The drawing under review shows one solid part. Ordinate dimensions are in mm from its lowest x, y, z. A direction names the side the tool comes from. Coordinates: 2 decimals unless noted, no trailing zeros. Write each loop counter-clockwise with the first axis right and the second up, starting at its lowest first coordinate (ties: lowest second). Pieces come first, ordered by that corner, then holes. Notation, with made-up numbers: M 75.25,15.5 L 90.25,15.5 A20 cw 90.25,54.5 Z; hole C 1,60.5 d9. An arc over 180 degrees is marked long. Write item = value, one per line.
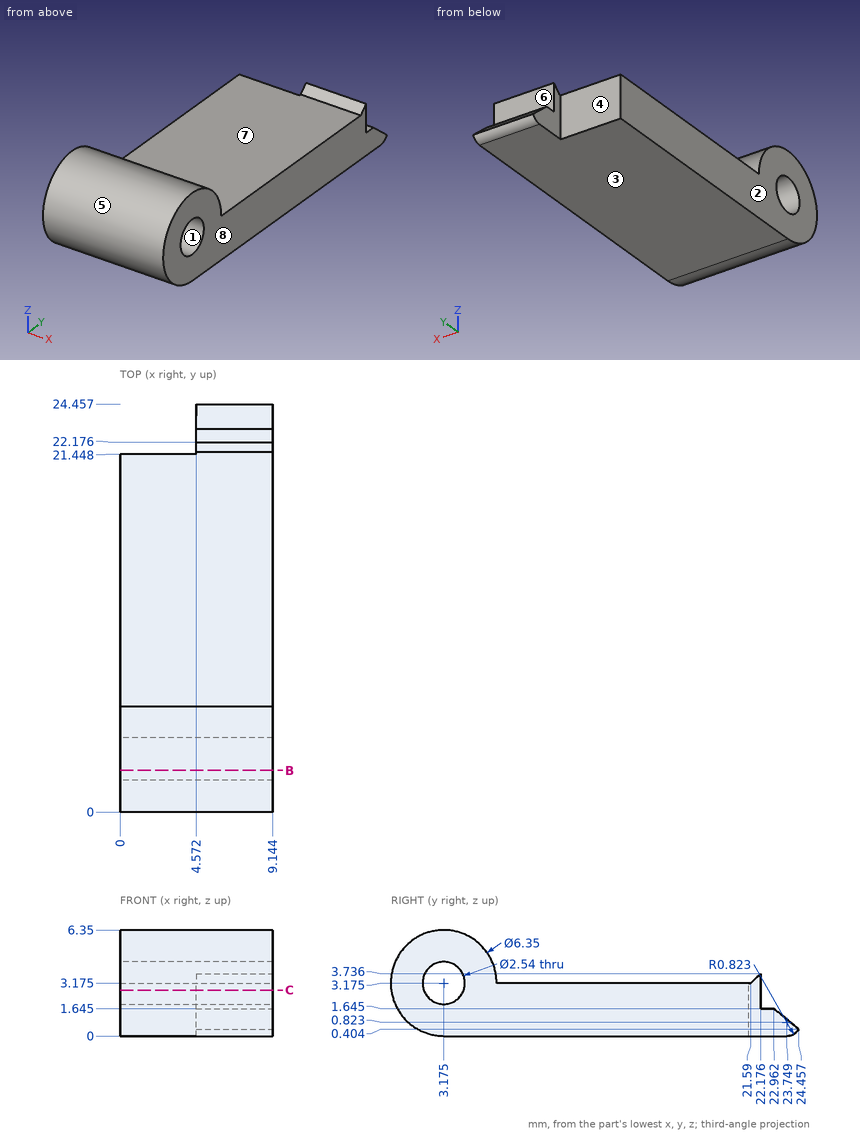
Q1. The part is to be moulded in two halves that separate along Z. For the marked faces 1, 2 and 3, say which applies: +Z half, -Z half, draft (parallel to the pull), parting line (faces both ways), or undercut.
Check result:
face_1 = undercut
face_2 = draft
face_3 = -Z half
Q2. Wall thickness on line 1 (X direction, y = 21.5, z = 1.25); line 2 (Z direction, x = 4.25, y = 13) (1 decimal); line 3 (Y direction, x = 7, z = 5.5) (1 decimal): over which ranges is each line inside the solid? List them lowest first.
Check result:
line_1 = 4.57 to 9.14
line_2 = 0 to 3.2
line_3 = 1 to 5.3
Q3. Consider section B-B, the plane y = 2.5. State the section outline as (x, z) points.
Check result:
outline = M 0,0.07 L 9.14,0.07 L 9.14,2.1 L 0,2.1 Z; M 0,4.25 L 9.14,4.25 L 9.14,6.28 L 0,6.28 Z
Q4. Machinability: for the marked faces 4, 5, 6, 7 and 8, which of the approach directions +Z, -Z, +X, -X, +Y, -Y give a long, thin tool a straight path to every point of the face, cutting with its end or side? Answer none if there is none.
Check result:
face_4 = +Z, -Z, -X, +Y
face_5 = +X, -X
face_6 = +Z, +X, -X, +Y
face_7 = +Z, +X, -X
face_8 = +Z, -Z, +X, +Y, -Y
Q5. For P1, Ø1.5, axis at y = 22.5, z = 1, coming from the -X side; P2, Ø3.5, axis at x = 3.5, z = 2, coming from the +Y side; P3, Ø0.6, axis at x = 6.5, z = 2.5, coming from the +Y side, all flat-tipped, find the tip position at first contact; note any pin that passes through.
Check result:
P1 = 4.57
P2 = 24.2
P3 = 22.18
Q6. Consider section C-C, the plane z = 2.75. State the section outline as (x, y) points (1 decimal).
Check result:
outline = M 0,0 L 9.1,0 L 9.1,2 L 0,2 Z; M 0,4.4 L 9.1,4.4 L 9.1,22.2 L 4.6,22.2 L 4.6,21.4 L 0,21.4 Z
